```python
from build123d import *

# Parameters (mm, degrees)
BOSS_EXTRUDE1_DEPTH = 5
SKETCH2_R           = 2
SKETCH2_R_2         = 1.5
SKETCH2_W           = 19
SKETCH2_H           = 40
SKETCH2_W_2         = 35
SKETCH2_H_2         = 16
SKETCH2_W_3         = 6
SKETCH2_H_3         = 8
CUT_EXTRUDE1_DEPTH  = 7
FILLET1_R           = 5
FILLET2_R           = 5
FILLET3_R           = 5
FILLET4_R           = 5
FILLET5_R           = 5
FILLET6_R           = 5
FILLET8_R           = 1
FILLET9_R           = 1
FILLET10_R          = 5


with BuildPart() as part:
    # Sketch1 → Boss-Extrude1 (new body)
    with BuildSketch(Plane(origin=(0, 0, 0), x_dir=(1, 0, 0), z_dir=(0, 1, 0))):
        Polygon((-16, 108), (16, 108), (16, 62), (52.5, 10), (52.5, -115), (-52.5, -115), (-52.5, 10), (-16, 62), align=None)
    extrude(amount=BOSS_EXTRUDE1_DEPTH)

    # Sketch2 → Cut-Extrude1 (cut)
    with BuildSketch(Plane(origin=(0, 5, 0), x_dir=(1, 0, 0), z_dir=(0, 1, 0))):
        with Locations(Location((-4.5, 103.5, 0), (0, 0, 270))):
            Circle(SKETCH2_R)
        with Locations(Location((4.5, 103.5, 0), (0, 0, 270))):
            Circle(SKETCH2_R)
        with Locations(Location((-5, 54.502551087, 0), (0, 0, 270))):
            Circle(SKETCH2_R)
        with Locations(Location((5, 54.502551087, 0), (0, 0, 270))):
            Circle(SKETCH2_R)
        with Locations(Location((-20.5, 48, 0), (0, 0, 270))):
            Circle(SKETCH2_R_2)
        with Locations(Location((20.5, 48, 0), (0, 0, 270))):
            Circle(SKETCH2_R_2)
        with Locations(Location((45.5, -6, 0), (0, 0, 270))):
            Circle(SKETCH2_R_2)
        with Locations(Location((-45.5, -6, 0), (0, 0, 270))):
            Circle(SKETCH2_R_2)
        with Locations(Location((45.5, -97, 0), (0, 0, 270))):
            Circle(SKETCH2_R_2)
        with Locations(Location((-45.5, -97, 0), (0, 0, 270))):
            Circle(SKETCH2_R_2)
        with Locations((0, 79)):
            Rectangle(SKETCH2_W, SKETCH2_H)
        with Locations((-35, -77)):
            Rectangle(SKETCH2_W_2, SKETCH2_H_2)
        with Locations((35, -77)):
            Rectangle(SKETCH2_W_2, SKETCH2_H_2)
        with Locations((-12, -78)):
            Rectangle(SKETCH2_W_3, SKETCH2_H_3)
        with Locations((12, -78)):
            Rectangle(SKETCH2_W_3, SKETCH2_H_3)
    extrude(amount=-CUT_EXTRUDE1_DEPTH, mode=Mode.SUBTRACT)

    # Fillet1
    fillet1_edges = [part.edges().sort_by_distance(p)[0] for p in [
        (16, 2.5, -108),
    ]]
    fillet(fillet1_edges, radius=FILLET1_R)

    # Fillet2
    fillet2_edges = [part.edges().sort_by_distance(p)[0] for p in [
        (-16, 2.5, -108),
    ]]
    fillet(fillet2_edges, radius=FILLET2_R)

    # Fillet3
    fillet3_edges = [part.edges().sort_by_distance(p)[0] for p in [
        (52.5, 2.5, -10),
    ]]
    fillet(fillet3_edges, radius=FILLET3_R)

    # Fillet4
    fillet4_edges = [part.edges().sort_by_distance(p)[0] for p in [
        (-52.5, 2.5, -10),
    ]]
    fillet(fillet4_edges, radius=FILLET4_R)

    # Fillet5
    fillet5_edges = [part.edges().sort_by_distance(p)[0] for p in [
        (52.5, 2.5, 115),
    ]]
    fillet(fillet5_edges, radius=FILLET5_R)

    # Fillet6
    fillet6_edges = [part.edges().sort_by_distance(p)[0] for p in [
        (-52.5, 2.5, 115),
    ]]
    fillet(fillet6_edges, radius=FILLET6_R)

    # Fillet8
    fillet8_edges = [part.edges().sort_by_distance(p)[0] for p in [
        (15, 2.5, 74),
    ]]
    fillet(fillet8_edges, radius=FILLET8_R)

    # Fillet9
    fillet9_edges = [part.edges().sort_by_distance(p)[0] for p in [
        (-15, 2.5, 82),
        (-15, 2.5, 74),
        (-9, 2.5, 74),
        (-9, 2.5, 82),
        (9, 2.5, 74),
        (15, 2.5, 82),
        (9, 2.5, 82),
    ]]
    fillet(fillet9_edges, radius=FILLET9_R)

    # Fillet10
    fillet10_edges = [part.edges().sort_by_distance(p)[0] for p in [
        (16, 2.5, -62),
        (-16, 2.5, -62),
    ]]
    fillet(fillet10_edges, radius=FILLET10_R)


solid = part.part
```
Part model, mm, in its own coordinate system. A direction names the side the tool comes from. Give positions to 0.01 mm unless a question says otherwise; leave off trailing zeros. Order: outer loops, then holes, each group sorted by start corner. A loop starts at its lowest first (then second) coordinate and runs counter-clockwise, first axis right, second up. Notation, with made-up numbers: (21, -3.5) - (67, -3.5) arc R28 cw to (67, 33.5) - close; hole circle Ø8 at (73, -38.5). An arc over 180 degrees is marked (long way). Use one line per item in the form item = value.
Item 1: Slice it at A-A on z = -87.5. Give the cut face in (x, y).
Solution:
outline = (-16, 0) - (-9.5, 0) - (-9.5, 5) - (-16, 5) - close; (9.5, 0) - (16, 0) - (16, 5) - (9.5, 5) - close
Item 2: Probe probe 1 along X at (y, z) = (1.4, 6); probe 2 along Z at (x, y) = (-1, 1.9); probe 3 along X at (y, z) = (3.3, -48). List the from-to ranges inside material, lowest first. Write a range as from..to.
Solution:
probe_1 = -52.5..-47, -44..44, 47..52.5
probe_2 = -108..-99, -59..115
probe_3 = -25.83..-22, -19..19, 22..25.83
Item 3: Slice it at C-C on y = 3.9. Count the separate pieces of the cut face and the enclosed holes in it, and give its area (3 significant figures).
Solution:
separate_pieces = 1
enclosed_holes = 13
area = 16,100 mm2
Item 4: Two-plate mould, pull along X, no slides. Class faces 1 (the face through (-3.899, 2.535, -101.592)), 2 (the face through (-14, 3, -107)), 3 (the face through (-35, 3, 85)): released by +X, released by -X, zero draft, split by the parting line, or undercut.
Solution:
face_1 = undercut
face_2 = released by -X
face_3 = zero draft
Item 5: Which spindle directions (+Z, -Z, +X, -X, +Y, -Y) get a long thin tool onto all of the face, cutting with end or side? Do faces 4 (the face through (-9, 3, 78)), 5 (the face through (-35, 3, 69)), 6 (the face through (17.5, 3, 77)), 7 (the face through (-51, 2.54, 113.57)), 8 (the face through (-52.5, 2, 31)). Say none if no direction does.
Solution:
face_4 = +Y, -Y
face_5 = -X, +Y, -Y
face_6 = +X, +Y, -Y
face_7 = +Z, -X, +Y, -Y
face_8 = +Z, -Z, -X, +Y, -Y
Item 6: Slice it at B-B on x = -27.5. Give the cut face in (y, z), and give its area (3 significant figures).
Solution:
outline = (0, -45.62) - (5, -45.62) - (5, 69) - (0, 69) - close; (0, 85) - (5, 85) - (5, 115) - (0, 115) - close
area = 723 mm2
Item 7: Pin check, flat tips, straight feed: pin 1 Ø1.5 at (y, z) = (2, 80.5) entering from -X; pin 2 Ø1 at (y, z) = (4, -81.5) entering from +X; pin 3 Ø1.5 at (y, z) = (1, -67.5) entering from -X. Stop position of each tip, or through.
Solution:
pin_1 = -17.5
pin_2 = 16
pin_3 = -16
Item 8: Slice it at D-D on z = -20. Give the cut face in (x, y), and give its area (3 significant figures).
Solution:
outline = (-45.48, 0) - (45.48, 0) - (45.48, 5) - (-45.48, 5) - close
area = 455 mm2
